Print and shaded views of the part. All mm, measured from the part's lowest x, y and z. A direction names the side the tool comes from. Round coordinates to 2 decimals unless told otherwise and drop trailing zeros. Loops run counter-clockwise (first coordinate to the right, second up) from the corner with the lowest first, then second, coordinate; pieces in that order, holes last. Notation, with made-up numbers: (-11, 57) - (24, 57) arc R27 cw to (24, 84) - close; hole circle Ø3 at (-22, -39). An arc over 180 degrees is marked (long way). Put each result on its own line as item: value. Start each with the question number.
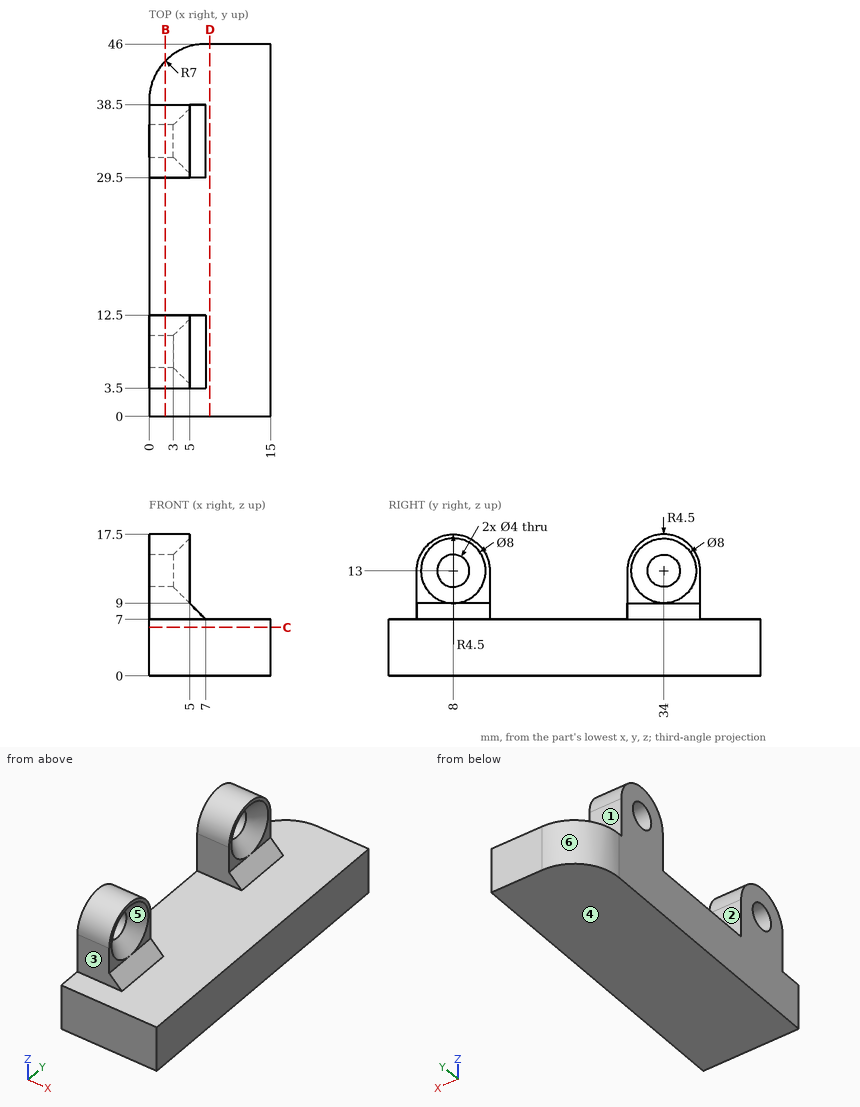
Item 1: Drill centre lines: probe 1 along Z at (x, y) = (0.6, 34); probe 2 along Y at (x, z) = (3.75, 12.25); probe 3 along Y at (x, z) = (2.75, 10.5). Where is each one in solid material? Low to high. Write a range as [from, to].
Item 2: Which spindle directions (+Z, -Z, +X, -X, +Y, -Y) get a long thin tool onto all of the face, cutting with end or side? Do the marked faces 1, 2 and 3. Say none if no direction does.
Item 3: Slice it at B-B (x = 2). Give the cut face in (y, z).
Item 4: Slice it at D-D (x = 7.5). Give the cut face in (y, z).
Item 5: Slice it at C-C (z = 6). Give the cut face in (x, y), plus the area to 4 significant figures.
Item 6: Two-plate mould, pull along Y, no slides. Class the marked faces 4, 5 and 6: pulls with the +Y half, pulls with the -Y half, needs draft (parallel to the pull), parting line crosses it, or undercut.
Item 7: Drop flat-ended pins along their axis: pin 1 Ø8 at (x, y) = (1.5, 29.5) entering from +Z; pin 2 Ø1.8 at (x, z) = (5, 9) entering from +Y; pin 3 Ø4.5 at (x, y) = (5.5, 28.5) entering from +Z; pin 4 Ø3.5 at (y, z) = (8, 13) entering from +X. Give the stop position or say it passes through.
Computed values:
1. probe 1: z = [0, 11], [15, 17.5]
1. probe 2: y = [3.5, 5.35], [10.65, 12.5], [29.5, 31.35], [36.65, 38.5]
1. probe 3: y = [3.5, 12.5], [29.5, 38.5]
2. face 1: +Z, +X, -X, +Y
2. face 2: +Z, +X, -X
2. face 3: +Z, +X, -X, -Y
3. outline: (0, 0) - (43.9, 0) - (43.9, 7) - (38.5, 7) - (38.5, 13) arc R4.5 ccw to (29.5, 13) - (29.5, 7) - (12.5, 7) - (12.5, 13) arc R4.5 ccw to (3.5, 13) - (3.5, 7) - (0, 7) - close; hole circle Ø4 at (8, 13); hole circle Ø4 at (34, 13)
4. outline: (0, 0) - (46, 0) - (46, 7) - (0, 7) - close
5. outline: (0, 0) - (15, 0) - (15, 46) - (7, 46) arc R7 ccw to (0, 39) - close
5. area: 679.5 mm^2
6. face 4: needs draft
6. face 5: undercut
6. face 6: pulls with the +Y half
7. pin 1: stops at z = 17.47
7. pin 2: stops at y = 38.5
7. pin 3: stops at z = 16.05
7. pin 4: passes through
